Input: dimensioned drawing with shaded views. Units: mm. Origin: part minimum x, y, z. A direction names the side the tool comes from. Round coordinates to 2 decimals unless told otherwise and drop trailing zeros. Loops run counter-clockwise (first coordinate to the right, second up) from the corner with the lowest first, then second, coordinate; pieces in that order, holes last. Notation, with made-up numbers: M 74,70 L 85,70 A20 cw 85,95 Z; hole C -17.75,-34.75 d4. An arc over 180 degrees is marked long. Write each question's results on one line, items separated by ' | '. Start each with the question number.
1. Section C-C on y = 15.5. Output: boundary loops of the cut face in (x, z).
2. Ray query, line 1 (Y direction, x = 14.5, z = 24.5); line 2 (X direction, y = 26.5, z = 28). Return the intervals inside material, ascending.
3. Section B-B on z = 15. Output: boundary loops of the cut face in (x, y), and give its area (3 significant figures).
4. Contact query for flat-ended pins moving along their axis: pin 1 Ø12 at (x, y) = (9.5, 8) entering from +Z; pin 2 Ø7.5 at (y, z) = (7.5, 6.5) entering from +X; pin 3 Ø1 at (x, z) = (10, 25) entering from +Y. Output: stop coordinate, or through.
5. Section A-A on x = 10. Output: boundary loops of the cut face in (y, z), and give its area (3 significant figures).
6. Set-up query: the marked faces 1, 2, 3 and 4. Return all of +Z, -Z, +X, -X, +Y, -Y with unobstructed straight access to the full face (end or side cutting, diameter ignored); none if empty.
7. Draft query along X for the marked faces 5, 6 and 7. Return one class per face: released by +X, released by -X, zero draft, split by the parting line, or undercut.
8. Section D-D on y = 9. Output: boundary loops of the cut face in (x, z).
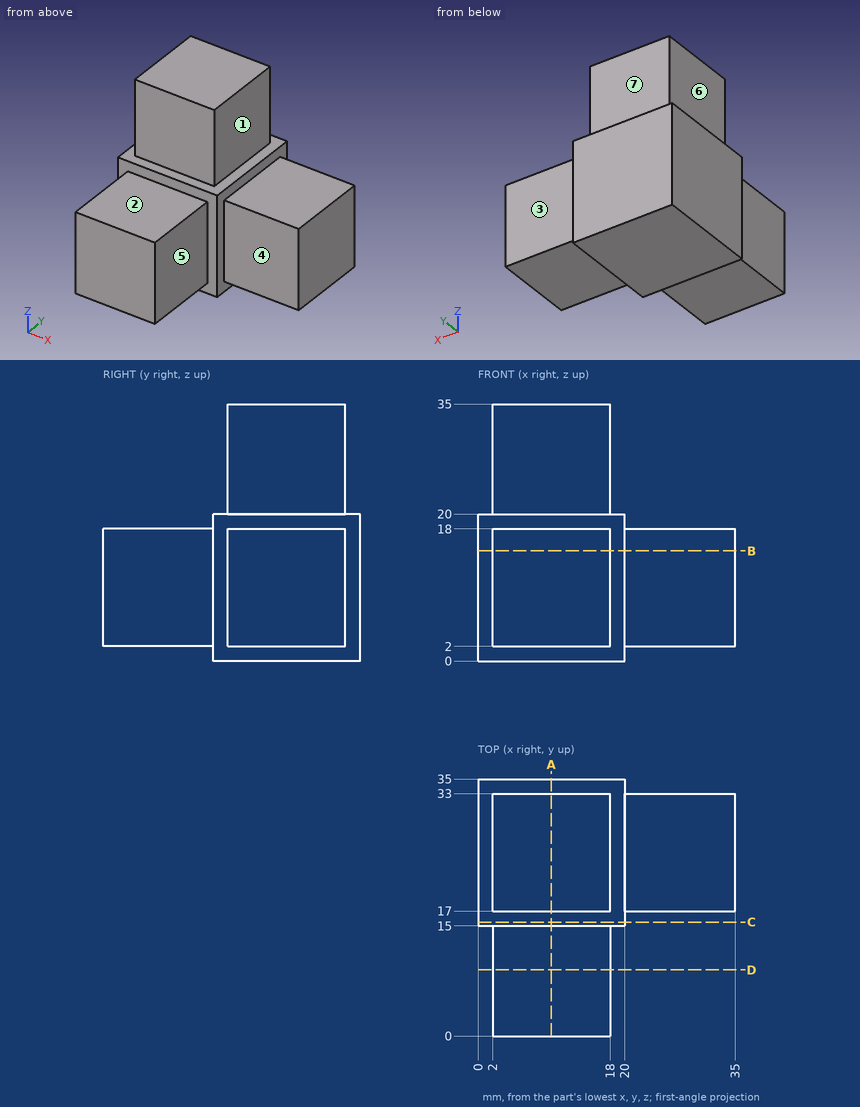
Taken from the geometry:
1) outline: M 0,0 L 20,0 L 20,20 L 0,20 Z
2) line 1: 17 to 33 | line 2: 2 to 18
3) outline: M 0,15 L 2,15 L 2,0 L 18,0 L 18,15 L 20,15 L 20,17 L 35,17 L 35,33 L 20,33 L 20,35 L 0,35 Z | area: 880 mm^2
4) pin 1: z = 18 | pin 2: x = 18 | pin 3: y = 33
5) outline: M 0,2 L 15,2 L 15,0 L 35,0 L 35,20 L 33,20 L 33,35 L 17,35 L 17,20 L 15,20 L 15,18 L 0,18 Z | area: 880 mm^2
6) face 1: +Z, +X, +Y, -Y | face 2: +Z, +X, -X, -Y | face 3: +Z, -Z, +X, +Y | face 4: +Z, -Z, +X, -Y
7) face 5: released by +X | face 6: released by -X | face 7: zero draft
8) outline: M 2,2 L 18,2 L 18,18 L 2,18 Z
